Autodesk Inventor part; units mm, degrees
ref_plane "YZ Plane" through (0, 0, 0) normal (1, 0, 0) x (0, 1, 0)
ref_plane "XZ Plane" through (0, 0, 0) normal (0, 1, 0) x (-1, 0, 0)
ref_plane "XY Plane" through (0, 0, 0) normal (0, 0, 1) x (1, 0, 0)
sketch "Sketch1" plane through (0, 0, 0) normal (0, 0, 1) x (1, 0, 0)
  line L0 (0, 0) -> (41.5036, 0)
  line L1 (41.5036, 0) -> (41.5036, 25.4)
  line L2 (41.5036, 25.4) -> (0, 25.4)
  line L3 (0, 25.4) -> (0, 0)
  dimension "d0" = 41.5036
  dimension "d1" = 25.4
extrude "Plate1" add sketch "Sketch1" along normal blind 3.048
sketch "Sketch3" plane through (0, 22.352, 0) normal (0, 1, 0) x (-1, 0, 0)
  line L0 (-41.5036, 0) -> (0, 0)
  line L1 (0, 0) -> (0, 25.4)
  line L2 (0, 25.4) -> (-41.5036, 25.4)
  line L3 (-41.5036, 25.4) -> (-41.5036, 0)
edge flange "Flange2" height 25.4 angle 90 thickness 3.048 bend radius 3.048 thickness toward (0, 1, 0) relief tear relief width 3.048 relief depth 1.524 edges at (20.7518, 25.4, 3.048) wall of the first edge with corners at (41.5036, 22.352, 0) (0, 22.352, 0) (0, 22.352, 25.4) (41.5036, 22.352, 25.4)
bend "Bend2"
corner "Corner2"
hole "Hole1" at (20.7518, 22.352, 15.748) direction (0, 1, 0) diameter 6.35 end through all
equation "\"d30\" = Thickness"
equation "\"d13\" = BendReliefWidth"
equation "\"d14\" = BendReliefDepth"
equation "\"d15\" = MinimumRemnant"
equation "\"d16\" = BendRadius"
equation "\"d19\" = BendRadius"
equation "\"d20\" = CornerReliefSize"
equation "\"d21\" = GapSize"
equation "\"d22\" = JacobiRadiusSize"
equation "\"BendRadius\" = Thickness"
equation "\"BendReliefWidth\" = Thickness"
equation "\"BendReliefDepth\" = 0.5 * Thickness"
equation "\"CornerReliefSize\" = 4 * Thickness"
equation "\"MinimumRemnant\" = 2 * Thickness"
equation "\"TransitionRadius\" = BendRadius"
equation "\"JacobiRadiusSize\" = BendRadius"
equation "\"GapSize\" = Thickness"
equation "\"d2\" = BendRadius"
properties part number "Chain Tension - L Bracket - Base"
Here's how the part is built. I have some questions about the finished solid (model axes, mm). A direction names the side the tool comes from. Give positions to 0.01 mm unless a question says otherwise; leave off trailing zeros. Loops run counter-clockwise (first coordinate to the right, second up) from the corner with the lowest first, then second, coordinate; pieces in that order, holes last. Notation, with made-up numbers: M -19,-28.75 L -4,-28.75 A18 cw -4,-17.75 Z; hole C -19,19 d9. An arc over 180 degrees is marked long. Use one line per item in the form item = value. Start each with the question number.
Q1. If we section it at D-D (x = 22.5): Write out the boundary of the cut face in (y, z).
Q2. If we section it at C-C (y = 23): Write out the boundary of the cut face in (x, z) (3 decimals), then the cut area to 3 significant figures.
Q3. Which directions (+Z, -Z, +X, -X, +Y, -Y) give clear straight access to the entire face, cutting with the end or side of a thin tool? Please do faces 5 (the flat face through (20, 10, 0)), 6 (the flat face through (20, 22.352, 11)).
Q4. If we section it at A-A (z = 17.5): Write out the boundary of the cut face in (x, y), then the cut area to 3 significant figures.
Q5. Will these pins go through, and if not, where does the flat tip stop? pin 1 Ø1.5 at (x, y) = (17, 7.5) entering from +Z; pin 2 Ø1 at (x, z) = (23.5, 6.5) entering from -Y; pin 3 Ø5.5 at (x, z) = (20.75, 15.75) entering from -Y.
Q6. I need wall thicknesses on line 1 along Y through (x, z) = (14, 21.75); line 2 along Z through (x, y) = (13.5, 7.25). Which ranges of each line are inside material? Lowest first, please.
Q7. If we section it at B-B (x = 28): Write out the boundary of the cut face in (y, z), then the cut area to 3 significant figures.
Q8. Thinking about a two-plate mould opening in X: for faces 1 (the cylindrical face through (20.61, 23.9, 18.92)), 2 (the flat face through (20, 24, 25.4)), 3 (the flat face through (0, 18, 2)), 4 (the flat face through (41.504, 18, 2)), which applies, +X half, -X half, draft (parallel to the pull), parting line (faces both ways), or undercut?
Taken from the geometry:
q1.outline = M 0,0 L 19.3,0 A6.1 ccw 25.4,6.1 L 25.4,13.1 L 22.35,13.1 L 22.35,6.1 A3.05 cw 19.3,3.05 L 0,3.05 Z; M 22.35,18.4 L 25.4,18.4 L 25.4,25.4 L 22.35,25.4 Z
q2.outline = M 0,1.248 L 41.504,1.248 L 41.504,25.4 L 0,25.4 Z; hole C 20.752,15.748 d6.35
q2.area = 971 mm^2
q3.face_5 = -Z, +X, -X, +Y, -Y
q3.face_6 = +Z, +X, -X, -Y
q4.outline = M 0,22.35 L 18.1,22.35 L 18.1,25.4 L 0,25.4 Z; M 23.4,22.35 L 41.5,22.35 L 41.5,25.4 L 23.4,25.4 Z
q4.area = 110 mm^2
q5.pin_1 = 3.05
q5.pin_2 = 22.35
q5.pin_3 = through
q6.line_1 = 22.35 to 25.4
q6.line_2 = 0 to 3.05
q7.outline = M 0,0 L 19.3,0 A6.1 ccw 25.4,6.1 L 25.4,25.4 L 22.35,25.4 L 22.35,6.1 A3.05 cw 19.3,3.05 L 0,3.05 Z
q7.area = 140 mm^2
q8.face_1 = undercut
q8.face_2 = draft
q8.face_3 = -X half
q8.face_4 = +X half
